Could you check a few things on this model? Use its own coordinates, in mm. Give positions to 0.01 mm unless a question says otherwise; leave off trailing zeros. Order: outer loops, then holes, each group sorted by start corner. A loop starts at its lowest first (then second) coordinate and runs counter-clockwise, first axis right, second up. Notation, with made-up numbers: (10, -27.75) -> (17, -27.75) arc R28 ccw to (17, 8.25) -> close; hole circle Ø9 at (40, 7.5). An arc over 180 degrees is marked (long way). Use one line per item in the form item = value. Start each with the question number.
from build123d import *

# Parameters (mm, degrees)
F0_W     = 200
F0_H     = 100
F1_DEPTH = 120


with BuildPart() as f1:
    # F0 (on Top) → F1 (new body)
    with BuildSketch(Plane.XY):
        with Locations((-2440, -1220)):
            Rectangle(F0_W, F0_H)
    extrude(amount=F1_DEPTH)

    # F2 (on face) → F3 (revolve)
    with BuildSketch(Plane.XZ.offset(1270)):
        with BuildLine():
            Line((-2380, 90.9458833933), (-2380, 30.9458833933))
            ThreePointArc((-2380, 30.9458833933), (-2350, 60.9458833933), (-2380, 90.9458833933))
        make_face()
    revolve(axis=Axis((-2380, -1270, 60.9458833933), (0, 0, -1)))

    # F5 (on face) → F8 section 0
    with BuildSketch(Plane(origin=(-2540, 0, 0), x_dir=(0, -1, 0), z_dir=(-1, 0, 0))):
        with BuildLine():
            add(Edge.make_bspline(
                [(1255, 60), (1255, 103.3012701892), (1202.5, 81.6506350946), (1150, 60), (1202.5, 38.3493649054), (1255, 16.6987298108), (1255, 60)],
                knots=[0, 0, 0, 2.0943951024, 2.0943951024, 4.1887902048, 4.1887902048, 6.2831853072, 6.2831853072, 6.2831853072], degree=2, weights=[1, 0.5, 1, 0.5, 1, 0.5, 1]))
        make_face()
    # F7 (on offset) → F8 section 1
    with BuildSketch(Plane(origin=(-2790, 0, 0), x_dir=(0, -1, 0), z_dir=(-1, 0, 0))):
        with BuildLine():
            add(Edge.make_bspline(
                [(1237.5, 60), (1237.5, 81.6506350946), (1211.25, 70.8253175473), (1185, 60), (1211.25, 49.1746824527), (1237.5, 38.3493649054), (1237.5, 60)],
                knots=[0, 0, 0, 2.0943951024, 2.0943951024, 4.1887902048, 4.1887902048, 6.2831853072, 6.2831853072, 6.2831853072], degree=2, weights=[1, 0.5, 1, 0.5, 1, 0.5, 1]))
        make_face()
    loft()


solid = f1.part
(1) Imagine slicing it at A-A (z = 101). Write out the boundary of the cut face in (x, y).
(2) Please list where these lines run through material, in increasing order: probe 1 along Y at (x, z) = (-2437.5, 19.5); probe 2 along X at (y, z) = (-1254.5, 103.5); probe 3 along Y at (x, z) = (-2644, 67).
(3) Imagine slicing it at D-D (x = -2374.5). Write out the boundary of the cut face in (y, z), plus the area to 3 significant figures.
(4) Imagine slicing it at C-C (y = -1279.5). Write out the boundary of the cut face in (x, z).
(5) I'm going to push flat-ended pins straight in: pin 1 Ø8 at (y, z) = (-1274.5, 32) entering from -X; pin 2 Ø1 at (x, z) = (-2558, 74) entering from +Y; pin 3 Ø4 at (x, z) = (-2549.5, 49.5) entering from +Y. Where does each tip first touch, or does it pass through?
(6) Imagine slicing it at B-B (x = -2424). Write out the boundary of the cut face in (y, z), plus the area to 3 significant figures.
Calculated:
q1.outline = (-2540, -1270) -> (-2340, -1270) -> (-2340, -1170) -> (-2540, -1170) -> close
q2.probe_1 = -1270 to -1170
q2.probe_2 = -2540 to -2340
q2.probe_3 = -1245.93 to -1194.07
q3.outline = (-1270, 0) -> (-1170, 0) -> (-1170, 120) -> (-1270, 120) -> (-1270, 90.44) arc R29.49 ccw to (-1270, 31.45) -> close
q3.area = 13,400 mm2
q4.outline = circle Ø56.91 at (-2380, 60.95)
q5.pin_1 = -2396.13
q5.pin_2 = -1192.05
q5.pin_3 = -1187.78
q6.outline = (-1270, 0) -> (-1170, 0) -> (-1170, 120) -> (-1270, 120) -> close
q6.area = 12,000 mm2
